The listing builds one solid part. Answer for the finished solid, in the listing's coordinates (mm). Face numbers are marked on the shaded views. A direction names the side the tool comes from. Coordinates: 2 decimals unless noted, no trailing zeros. Loops run counter-clockwise (first coordinate to the right, second up) from the corner with the lowest first, then second, coordinate; pieces in that order, holes last. Notation, with made-up numbers: (80.5, 38.5) - (85.5, 38.5) arc R30 ccw to (85.5, 65.5) - close; hole circle Ø2 at (66, 13). An arc over 180 degrees is marked (long way). Return JSON: item names as keys, results as strings. Group by question number.
1. This flat-tipped pin is pushed along its axis until it touches: P1, Ø1.5, axis at x = -3.5, y = 8, coming from the +Z side. Where does it stop, or does it pass through?
2. Section A-A (y = 0) is taken. Write down the section's boundary in (x, z), and give its area (4 significant figures).
3. Find the intervals of material crossed by line 1 along Y through (x, z) = (4.5, -0.9); line 2 along Y through (x, z) = (0, -1.1); line 3 along X through (y, z) = (-7.75, -1.6), in increasing order.
4. Section D-D (x = -3.25) is taken. Write down the section's boundary in (y, z).
5. Which of the six approach directions +Z, -Z, +X, -X, +Y, -Y give full straight-line access (tool end or side, diameter ignored) to the marked faces 4 and 5?
6. The mould has two halves that part along Y. Classify the marked faces 1, 2 and 3: pulls with the +Y half, pulls with the -Y half, needs draft (parallel to the pull), parting line crosses it, or undercut.
7. Section C-C (x = 0) is taken. Write down the section's boundary in (y, z), and give its area (3 significant figures).
8. Section B-B (z = -1.8) is taken. Write down the section's boundary in (x, y).
```python
from build123d import *

# Parameters (mm, degrees)
SKETCH001_W     = 15
SKETCH001_H     = 20
PAD_DEPTH       = 3
SKETCH_R        = 4.5
POCKET_DEPTH    = 3
SKETCH002_W     = 2
SKETCH002_H     = 4
POCKET001_DEPTH = 3
POCKET002_DEPTH = 3


with BuildPart() as part:
    # Sketch001 → Pad (new body)
    with BuildSketch(Plane.XY):
        Rectangle(SKETCH001_W, SKETCH001_H)
    extrude(amount=-PAD_DEPTH)

    # Sketch → Pocket (cut)
    with BuildSketch(Plane.XY):
        Circle(SKETCH_R)
    extrude(amount=-POCKET_DEPTH, mode=Mode.SUBTRACT)

    # Sketch002 (on Face4 of Pocket) → Pocket001 (cut)
    with BuildSketch(Plane.XY):
        with Locations((3.55, 0)):
            Rectangle(SKETCH002_W, SKETCH002_H)
    extrude(amount=-POCKET001_DEPTH, mode=Mode.SUBTRACT)

    # Sketch003 (on Face4 of Pocket001) → Pocket002 (cut)
    with BuildSketch(Plane.XY):
        Polygon((3.05, -11), (-3.5, -11), (-4, 0), (3.55, 0), align=None)
    extrude(amount=-POCKET002_DEPTH, mode=Mode.SUBTRACT)


solid = part.part
```
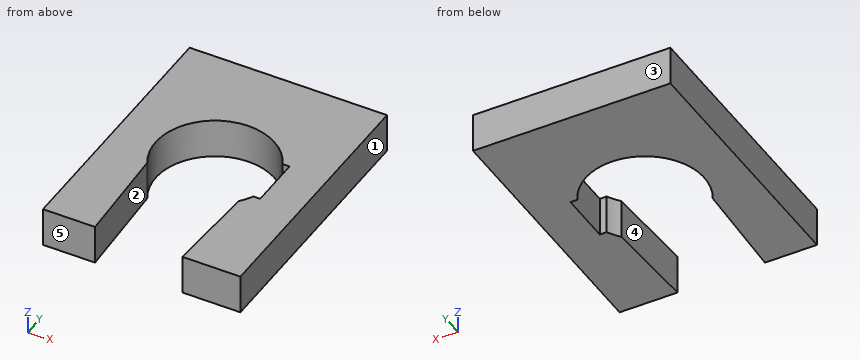
The answers:
{
 "1": {"P1": "stops at z = 0"},
 "2": {"outline": "(-7.5, -3) - (-4.5, -3) - (-4.5, 0) - (-7.5, 0) - close; (4.55, -3) - (7.5, -3) - (7.5, 0) - (4.55, 0) - close", "area": "17.85 mm2"},
 "3": {"line 1": "y = -10 to -2, 2 to 10", "line 2": "y = 4.5 to 10", "line 3": "x = -7.5 to -3.65, 3.2 to 7.5"},
 "4": {"outline": "(3.11, -3) - (10, -3) - (10, 0) - (3.11, 0) - close"},
 "5": {"face 4": "+Z, -Z", "face 5": "+Z, -Z, +X, -X, -Y"},
 "6": {"face 1": "needs draft", "face 2": "undercut", "face 3": "pulls with the +Y half"},
 "7": {"outline": "(4.5, -3) - (10, -3) - (10, 0) - (4.5, 0) - close", "area": "16.5 mm2"},
 "8": {"outline": "(-7.5, -10) - (-3.55, -10) - (-3.9, -2.25) arc R4.5 cw (long way) to (4.03, 2) - (4.55, 2) - (4.55, -2) - (4.03, -2) arc R4.5 cw to (3.42, -2.93) - (3.1, -10) - (7.5, -10) - (7.5, 10) - (-7.5, 10) - close"}
}
